```python
from build123d import *

# Parameters (mm, degrees)
F3_W      = 50
F3_H      = 105
F4_DEPTH  = 2
F5_W      = 50
F5_H      = 105
F5_W_2    = 46
F5_H_2    = 101
F6_DEPTH  = 26
F7_R      = 2.5
F8_R      = 8.25
F9_DEPTH  = 2
F10_R     = 5.25
F11_DEPTH = 2
F13_W     = 6
F13_H     = 1
F13_W_2   = 1
F13_H_2   = 6.5
F13_H_3   = 68
F13_W_3   = 40
F14_DEPTH = 18
F15_W     = 40
F15_H     = 1
F16_DEPTH = 6
F18_DEPTH = 6
F19_R     = 1.55
F20_DEPTH = 2.2
F12_R     = 11
F21_DEPTH = 1


with BuildPart() as f4:
    # F3 (on Top) → F4 (new body)
    with BuildSketch(Plane.XY):
        Rectangle(F3_W, F3_H)
    extrude(amount=F4_DEPTH)

    # F5 (on face) → F6 (join)
    with BuildSketch(Plane.XY.offset(2)):
        Rectangle(F5_W, F5_H)
        Rectangle(F5_W_2, F5_H_2, mode=Mode.SUBTRACT)
    extrude(amount=F6_DEPTH)

    # F7
    f7_edges = [f4.edges().sort_by_distance(p)[0] for p in [
        (-25, 52.5, 14),
        (25, 52.5, 14),
        (25, -52.5, 14),
        (-25, -52.5, 14),
    ]]
    fillet(f7_edges, radius=F7_R)

    # F8 (on face) → F9 (cut)
    with BuildSketch(Plane(origin=(-25, 0, 0), x_dir=(0, -1, 0), z_dir=(-1, 0, 0))):
        with Locations((-36.5, 15)):
            Circle(F8_R)
    extrude(amount=-F9_DEPTH, mode=Mode.SUBTRACT)

    # F10 (on face) → F11 (cut)
    with BuildSketch(Plane(origin=(0, 52.5, 0), x_dir=(-1, 0, 0), z_dir=(0, 1, 0))):
        with Locations((0, 15)):
            Circle(F10_R)
    extrude(amount=-F11_DEPTH, mode=Mode.SUBTRACT)

    # F13 (on face) → F14 (join)
    with BuildSketch(Plane.XY.offset(2)):
        with Locations((20, 20)):
            Rectangle(F13_W, F13_H)
        with Locations((20, -49)):
            Rectangle(F13_W, F13_H)
        Polygon((10, 20.5), (-3, 20.5), (-3, 19.5), (3, 19.5), (4, 19.5), (10, 19.5), align=None)
        with Locations((3.5, 16.25)):
            Rectangle(F13_W_2, F13_H_2)
        Polygon((-3, -48.5), (-3, -49.5), (10, -49.5), (10, -48.5), (4, -48.5), (3, -48.5), align=None)
        with Locations((3.5, -45.25)):
            Rectangle(F13_W_2, F13_H_2)
        Polygon((-10, 19.5), (-10, 20.5), (-17, 20.5), (-17, 19.5), (-16, 19.5), align=None)
        with Locations((-16.5, -14.5)):
            Rectangle(F13_W_2, F13_H_3)
        Polygon((-16, -48.5), (-17, -48.5), (-17, -49.5), (-10, -49.5), (-10, -48.5), align=None)
        with Locations((3, 22)):
            Rectangle(F13_W_3, F13_H)
    extrude(amount=F14_DEPTH)

    # F15 (on face) → F16 (join)
    with BuildSketch(Plane.XY.offset(2)):
        with Locations((3, 21)):
            Rectangle(F15_W, F15_H)
        with Locations((3, -50)):
            Rectangle(F15_W, F15_H)
    extrude(amount=F16_DEPTH)

    # F17 (on face) → F18 (join)
    with BuildSketch(Plane.XY.offset(20)):
        with BuildLine():
            Line((-23, 46.5), (-20.5, 46.5))
            ThreePointArc((-20.5, 46.5), (-19.4393398282, 46.9393398282), (-19, 48))
            Line((-19, 48), (-19, 50.5))
            Line((-19, 50.5), (-23, 50.5))
            Line((-23, 50.5), (-23, 46.5))
        make_face()
        with BuildLine():
            ThreePointArc((19, 48), (19.4393398282, 46.9393398282), (20.5, 46.5))
            Line((20.5, 46.5), (23, 46.5))
            Line((23, 46.5), (23, 50.5))
            Line((23, 50.5), (19, 50.5))
            Line((19, 50.5), (19, 48))
        make_face()
        with BuildLine():
            ThreePointArc((20.5, -46.5), (19.4393398282, -46.9393398282), (19, -48))
            Line((19, -48), (19, -50.5))
            Line((19, -50.5), (23, -50.5))
            Line((23, -50.5), (23, -46.5))
            Line((23, -46.5), (20.5, -46.5))
        make_face()
        with BuildLine():
            ThreePointArc((-19, -48), (-19.4393398282, -46.9393398282), (-20.5, -46.5))
            Line((-20.5, -46.5), (-23, -46.5))
            Line((-23, -46.5), (-23, -50.5))
            Line((-23, -50.5), (-19, -50.5))
            Line((-19, -50.5), (-19, -48))
        make_face()
    extrude(amount=F18_DEPTH)

    # F19 (on face) → F20 (cut)
    with BuildSketch(Plane.XY.offset(26)):
        with Locations((-21, 48.5)):
            Circle(F19_R)
        with Locations((21, 48.5)):
            Circle(F19_R)
        with Locations((-21, -48.5)):
            Circle(F19_R)
        with Locations((21, -48.5)):
            Circle(F19_R)
    extrude(amount=-F20_DEPTH, mode=Mode.SUBTRACT)

    # F12 (on face) → F21 (cut)
    with BuildSketch(Plane(origin=(0, 52.5, 0), x_dir=(-1, 0, 0), z_dir=(0, 1, 0))):
        with Locations((0, 15)):
            Circle(F12_R)
    extrude(amount=-F21_DEPTH, mode=Mode.SUBTRACT)


solid = f4.part
```
CAD build for the part. Positions are in the model's coordinates, mm. A direction names the side the tool comes from. Coordinates: 2 decimals unless noted, no trailing zeros. Loops run counter-clockwise (first coordinate to the right, second up) from the corner with the lowest first, then second, coordinate; pieces in that order, holes last. Notation, with made-up numbers: (74.25, -35.5) - (126.25, -35.5) arc R18 cw to (126.25, -10.5) - close; hole circle Ø9 at (30.25, -37). An arc over 180 degrees is marked (long way). Return JSON: item names as keys, results as strings.
1. Band-saw the part on C-C (y = -24). Give the cut face in (x, z).
Result:
{"outline": "(-25, 0) - (25, 0) - (25, 28) - (23, 28) - (23, 2) - (-16, 2) - (-16, 20) - (-17, 20) - (-17, 2) - (-23, 2) - (-23, 28) - (-25, 28) - close"}
2. Band-saw the part on D-D (z = 15). State how many separate pieces and enclosed holes the cut face has, and give its area (3 significant figures).
Result:
{"separate pieces": "5", "enclosed holes": "0", "area": "706 mm2"}
3. 3-axis set-ups, long thin cutter, end or side, ignore diameter. For faces 5 (the flat face through (3, -45, 11)), 6 (the flat face through (24, 16, 28)), 7 (the flat face through (20, -49.5, 14)): which of +Z, -Z, +X, -X, +Y, -Y reach the whole face in a straight line?
Result:
{"face 5": "+Z", "face 6": "+Z, +X, -X, +Y, -Y", "face 7": "none"}
4. Probe L1, parallel to X at y = 8.5, z = 18; L2, parallel to Y at x = 5.5, z = 6; L3, parallel to Y at x = -10.5, z = 13. List the from-to ranges inside material, lowest first. Write a range as from..to.
Result:
{"L1": "x = -25..-23, -17..-16, 23..25", "L2": "y = -52.5..-48.5, 19.5..22.5, 50.5..51.5", "L3": "y = -52.5..-50.5, -49.5..-48.5, 19.5..20.5, 21.5..22.5, 50.5..51.5"}
5. Band-saw the part on A-A (x = 0). Give the cut face in (y, z), and give its area (4 significant figures).
Result:
{"outline": "(-52.5, 0) - (52.5, 0) - (52.5, 4) - (51.5, 4) - (51.5, 9.75) - (50.5, 9.75) - (50.5, 2) - (22.5, 2) - (22.5, 20) - (21.5, 20) - (21.5, 8) - (20.5, 8) - (20.5, 20) - (19.5, 20) - (19.5, 2) - (-48.5, 2) - (-48.5, 20) - (-49.5, 20) - (-49.5, 8) - (-50.5, 8) - (-50.5, 28) - (-52.5, 28) - close; (50.5, 20.25) - (51.5, 20.25) - (51.5, 26) - (52.5, 26) - (52.5, 28) - (50.5, 28) - close", "area": "347.5 mm2"}
6. Mould opens along Y. For faces 1 (the flat face through (4, 20.5, 14)), 2 (the flat face through (-7, 20.5, 5)), 3 (the cylindrical face through (-24, -52, 14)), 4 (the flat face through (-5, 52.5, 4)) say: released by +Y, released by -Y, zero draft, split by the parting line, or undercut.
Result:
{"face 1": "undercut", "face 2": "undercut", "face 3": "released by -Y", "face 4": "released by +Y"}
7. Drop flat-ended pins along their axis: pin 1 (9 mm diameter, centred on x = -2, z = 10, fed in from +Y); pin 2 (4 mm diameter, centred on x = 4.5, y = -17, fed in from -Z). Give the stop position or say it passes through.
Result:
{"pin 1": "stops at y = 51.5", "pin 2": "stops at z = 0"}
8. Band-saw the part on B-B (y = 42). Give the cut face in (x, z), and give its area (3 significant figures).
Result:
{"outline": "(-25, 0) - (25, 0) - (25, 28) - (23, 28) - (23, 2) - (-23, 2) - (-23, 8.85) - (-25, 8.85) - close; (-25, 21.15) - (-23, 21.15) - (-23, 28) - (-25, 28) - close", "area": "179 mm2"}
